```python
from build123d import *

# Parameters (mm, degrees)
BOSS_EXTRUDE1_DEPTH = 6.35
SHELL1_T            = -1.524
SKETCH2_W           = 53.975
SKETCH2_H           = 53.975
BOSS_EXTRUDE2_DEPTH = 0.762
SKETCH3_W           = 2.54
SKETCH3_H           = 9.525
CUT_EXTRUDE1_DEPTH  = 172.008977963
SKETCH4_R           = 6.2865
SKETCH4_R_2         = 4.7625
BOSS_EXTRUDE3_DEPTH = 4.826
RIB1_REACH          = 173.009
SKETCH5_WALLS_W     = 437.807455926
SKETCH5_WALLS_H     = 1.27
SKETCH5_WALLS_W_2   = 1.27
SKETCH5_WALLS_H_2   = 437.807455926


with BuildPart() as part:
    # Sketch1 → Boss-Extrude1 (new body)
    with BuildSketch(Plane.XY):
        with BuildLine():
            Line((101.6, 101.6), (107.95, 101.6))
            ThreePointArc((107.95, 101.6), (112.440128061, 99.740128061), (114.3, 95.25))
            Line((114.3, 95.25), (114.3, 82.55))
            ThreePointArc((114.3, 82.55), (112.440128061, 78.059871939), (107.95, 76.2))
            Line((107.95, 76.2), (104.775, 76.2))
            ThreePointArc((104.775, 76.2), (102.52993597, 75.27006403), (101.6, 73.025))
            Line((101.6, 73.025), (101.6, -95.25))
            ThreePointArc((101.6, -95.25), (99.740128061, -99.740128061), (95.25, -101.6))
            Line((95.25, -101.6), (62.217039467, -101.6))
            ThreePointArc((62.217039467, -101.6), (57.416890659, -102.542084733), (53.328890971, -105.228571429))
            ThreePointArc((53.328890971, -105.228571429), (0, -127), (-53.328890971, -105.228571429))
            ThreePointArc((-53.328890971, -105.228571429), (-57.416890659, -102.542084733), (-62.217039467, -101.6))
            Line((-62.217039467, -101.6), (-95.25, -101.6))
            ThreePointArc((-95.25, -101.6), (-99.740128061, -99.740128061), (-101.6, -95.25))
            Line((-101.6, -95.25), (-101.6, 95.25))
            ThreePointArc((-101.6, 95.25), (-99.740128061, 99.740128061), (-95.25, 101.6))
            Line((-95.25, 101.6), (101.6, 101.6))
        make_face()
        with BuildLine():
            Line((-34.454236314, -101.6), (34.454236314, -101.6))
            ThreePointArc((34.454236314, -101.6), (36.890518728, -103.42157951), (35.832405767, -106.2736))
            ThreePointArc((35.832405767, -106.2736), (0, -116.84), (-35.832405767, -106.2736))
            ThreePointArc((-35.832405767, -106.2736), (-36.890518728, -103.42157951), (-34.454236314, -101.6))
        make_face(mode=Mode.SUBTRACT)
    extrude(amount=BOSS_EXTRUDE1_DEPTH)

    # Shell1
    shell1_openings = [part.faces().sort_by_distance(p)[0] for p in [
        (0.794834734, -2.433656068, 0),
    ]]
    offset(amount=SHELL1_T, openings=shell1_openings, kind=Kind.INTERSECTION)

    # Sketch2 → Boss-Extrude2 (add)
    with BuildSketch(Plane.XY.offset(6.35)):
        with Locations((68.58, 0)):
            Rectangle(SKETCH2_W, SKETCH2_H)
        Rectangle(SKETCH2_W, SKETCH2_H)
        with Locations((68.58, 68.58)):
            Rectangle(SKETCH2_W, SKETCH2_H)
        with Locations((68.58, -68.58)):
            Rectangle(SKETCH2_W, SKETCH2_H)
        with Locations((0, -68.58)):
            Rectangle(SKETCH2_W, SKETCH2_H)
        with Locations((-68.58, -68.58)):
            Rectangle(SKETCH2_W, SKETCH2_H)
        with Locations((-68.58, 0)):
            Rectangle(SKETCH2_W, SKETCH2_H)
        with Locations((-68.58, 68.58)):
            Rectangle(SKETCH2_W, SKETCH2_H)
        with Locations((0, 68.58)):
            Rectangle(SKETCH2_W, SKETCH2_H)
    extrude(amount=BOSS_EXTRUDE2_DEPTH)

    # Sketch3 → Cut-Extrude1 (cut, through all)
    with BuildSketch(Plane.XY.offset(7.112)):
        with Locations((-81.28, 93.6625)):
            Rectangle(SKETCH3_W, SKETCH3_H)
        with Locations((-76.2, 93.6625)):
            Rectangle(SKETCH3_W, SKETCH3_H)
        with Locations((76.2, 93.6625)):
            Rectangle(SKETCH3_W, SKETCH3_H)
        with Locations((81.28, 93.6625)):
            Rectangle(SKETCH3_W, SKETCH3_H)
        with Locations((81.28, -93.6625)):
            Rectangle(SKETCH3_W, SKETCH3_H)
        with Locations((76.2, -93.6625)):
            Rectangle(SKETCH3_W, SKETCH3_H)
        with Locations((-76.2, -93.6625)):
            Rectangle(SKETCH3_W, SKETCH3_H)
        with Locations((-81.28, -93.6625)):
            Rectangle(SKETCH3_W, SKETCH3_H)
    extrude(amount=-CUT_EXTRUDE1_DEPTH, mode=Mode.SUBTRACT)

    # Sketch4 → Boss-Extrude3 (add)
    with BuildSketch(Plane(origin=(0, 0, 4.826), x_dir=(-1, 0, 0), z_dir=(0, 0, -1))):
        Circle(SKETCH4_R)
        Circle(SKETCH4_R_2, mode=Mode.SUBTRACT)
    extrude(amount=BOSS_EXTRUDE3_DEPTH)

    # Sketch5 walls → Rib1 (add, up to next)
    with BuildSketch(Plane(origin=(0, 0, 0), x_dir=(-1, 0, 0), z_dir=(0, 0, -1)), mode=Mode.PRIVATE) as rib1_sk1:
        with Locations((53.18125, 0)):
            Rectangle(SKETCH5_WALLS_W, SKETCH5_WALLS_H)
    rib1_tool1 = extrude(rib1_sk1.sketch, amount=-RIB1_REACH, mode=Mode.PRIVATE) - part.part
    # Sketch5 walls → Rib1 (add, up to next)
    with BuildSketch(Plane(origin=(0, 0, 0), x_dir=(-1, 0, 0), z_dir=(0, 0, -1)), mode=Mode.PRIVATE) as rib1_sk2:
        with Locations((-53.18125, 0)):
            Rectangle(SKETCH5_WALLS_W, SKETCH5_WALLS_H)
    rib1_tool2 = extrude(rib1_sk2.sketch, amount=-RIB1_REACH, mode=Mode.PRIVATE) - part.part
    # Sketch5 walls → Rib1 (add, up to next)
    with BuildSketch(Plane(origin=(0, 0, 0), x_dir=(-1, 0, 0), z_dir=(0, 0, -1)), mode=Mode.PRIVATE) as rib1_sk3:
        with Locations((0, -53.18125)):
            Rectangle(SKETCH5_WALLS_W_2, SKETCH5_WALLS_H_2)
    rib1_tool3 = extrude(rib1_sk3.sketch, amount=-RIB1_REACH, mode=Mode.PRIVATE) - part.part
    # Sketch5 walls → Rib1 (add, up to next)
    with BuildSketch(Plane(origin=(0, 0, 0), x_dir=(-1, 0, 0), z_dir=(0, 0, -1)), mode=Mode.PRIVATE) as rib1_sk4:
        with Locations((0, 53.18125)):
            Rectangle(SKETCH5_WALLS_W_2, SKETCH5_WALLS_H_2)
    rib1_tool4 = extrude(rib1_sk4.sketch, amount=-RIB1_REACH, mode=Mode.PRIVATE) - part.part
    # Sketch5 walls → Rib1 (add, up to next)
    with BuildSketch(Plane(origin=(0, 0, 0), x_dir=(-1, 0, 0), z_dir=(0, 0, -1)), mode=Mode.PRIVATE) as rib1_sk5:
        Polygon((-116.734475157, -117.632500769), (220.740224875, 219.842199263), (219.842199263, 220.740224875), (-117.632500769, -116.734475157), align=None)
    rib1_tool5 = extrude(rib1_sk5.sketch, amount=-RIB1_REACH, mode=Mode.PRIVATE) - part.part
    # Sketch5 walls → Rib1 (add, up to next)
    with BuildSketch(Plane(origin=(0, 0, 0), x_dir=(-1, 0, 0), z_dir=(0, 0, -1)), mode=Mode.PRIVATE) as rib1_sk6:
        Polygon((-117.632500769, 116.734475157), (219.842199263, -220.740224875), (220.740224875, -219.842199263), (-116.734475157, 117.632500769), align=None)
    rib1_tool6 = extrude(rib1_sk6.sketch, amount=-RIB1_REACH, mode=Mode.PRIVATE) - part.part
    # Sketch5 walls → Rib1 (add, up to next)
    with BuildSketch(Plane(origin=(0, 0, 0), x_dir=(-1, 0, 0), z_dir=(0, 0, -1)), mode=Mode.PRIVATE) as rib1_sk7:
        Polygon((116.734475157, 117.632500769), (-220.740224875, -219.842199263), (-219.842199263, -220.740224875), (117.632500769, 116.734475157), align=None)
    rib1_tool7 = extrude(rib1_sk7.sketch, amount=-RIB1_REACH, mode=Mode.PRIVATE) - part.part
    # Sketch5 walls → Rib1 (add, up to next)
    with BuildSketch(Plane(origin=(0, 0, 0), x_dir=(-1, 0, 0), z_dir=(0, 0, -1)), mode=Mode.PRIVATE) as rib1_sk8:
        Polygon((117.632500769, -116.734475157), (-221.255701937, 222.153727549), (-222.153727549, 221.255701937), (116.734475157, -117.632500769), align=None)
    rib1_tool8 = extrude(rib1_sk8.sketch, amount=-RIB1_REACH, mode=Mode.PRIVATE) - part.part
    add(rib1_tool1.solids().sort_by_distance((-53.18125, 0, 0))[0])
    add(rib1_tool2.solids().sort_by_distance((53.18125, 0, 0))[0])
    add(rib1_tool3.solids().sort_by_distance((0, -53.18125, 0))[0])
    add(rib1_tool4.solids().sort_by_distance((0, 53.18125, 0))[0])
    add(rib1_tool5.solids().sort_by_distance((-51.553862053, 51.553862053, 0))[0])
    add(rib1_tool6.solids().sort_by_distance((-51.553862053, -51.553862053, 0))[0])
    add(rib1_tool7.solids().sort_by_distance((51.553862053, -51.553862053, 0))[0])
    add(rib1_tool8.solids().sort_by_distance((52.26061339, 52.26061339, 0))[0])


solid = part.part
```
For this review, take the finished solid that the model builds, in its own axes (mm). A direction names the side the tool comes from. Coordinates: 2 decimals unless noted, no trailing zeros. Use one line per item in the form item = value. Start each with the question number.
1) Take a section at A-A (z = 3.25). State how many separate pieces and enclosed holes the cut face has, plus the area to 3 significant figures.
2) For faces 1 (the face through (68, -68, 7.112)), 2 (the face through (38.33, -102.92, 2.38)), list the 3-axis set-ups (+Z, -Z, +X, -X, +Y, -Y) from which the entire face can be reached by the end or side of a thin tool; tool diameter is ignored.
3) Draft analysis for pull direction X (two halves, no side actions). For faces 3 (the face through (-99.79, 99.69, 3.13)), 4 (the face through (57.481, -102.516, 3.131)), 5 (the face through (111.325, 98.7, 2.379)), 6 (the face through (0, 0, 7.112)), state which applies: released by +X, released by -X, zero draft, split by the parting line, or undercut.
4) To check wall thickness, follow probe 1 along X at (y, z) = (4, 7); probe 2 along X at (y, z) = (90, 5.25); probe 3 along Y at (x, z) = (-59.5, 2.5) (3 decimals). State the ranges of each line that lie inside material, in increasing order. Write a range as from..to.
5) For pin 1 (1.2 mm diameter, centred on x = 81, z = 6, fed in from -Y); pin 2 (0.8 mm diameter, centred on x = 92, z = 7, fed in from +Y); pin 3 (0.8 mm diameter, centred on x = 57, z = 6.5, fed in from -Y), all flat-tipped, find the tip position at first contact; note any pin that passes through.
From the geometry:
q1.separate_pieces = 1
q1.enclosed_holes = 9
q1.area = 2,720 mm2
q2.face_1 = +Z, +X, -X, +Y, -Y
q2.face_2 = -Z
q3.face_3 = released by -X
q3.face_4 = released by +X
q3.face_5 = undercut
q3.face_6 = zero draft
q4.probe_1 = -95.57..-41.59, -26.99..26.99, 41.59..95.57
q4.probe_2 = -101.6..-82.55, -80.01..-77.47, -74.93..74.93, 77.47..80.01, 82.55..114.3
q4.probe_3 = -101.894..-100.338, -60.398..-58.602, -0.635..0.635, 58.602..60.398, 100.076..101.6
q5.pin_1 = -101.6
q5.pin_2 = 95.57
q5.pin_3 = -102.9
